```python
from build123d import *

# Parameters (mm, degrees)
F0_W     = 76.2
F0_H     = 203.2
F1_DEPTH = 6.35
F3_D     = 6.35
F5_D     = 19.05
F7_D     = 34.925


with BuildPart() as f1:
    # F0 (on Front) → F1 (new body)
    with BuildSketch(Plane.XZ):
        with Locations((38.1, 101.6)):
            Rectangle(F0_W, F0_H)
    extrude(amount=F1_DEPTH)

    # F3 (through all)
    with Locations(Plane.XZ.offset(6.35)):
        with Locations((13.868812, 74.729279), (61.493812, 74.729279), (61.493812, 27.104279), (13.868812, 27.104279)):
            Hole(F3_D / 2)

    # F5 (through all)
    with Locations(Plane.XZ.offset(6.35)):
        with Locations((38.1, 173.591416)):
            Hole(F5_D / 2)

    # F7 (through all)
    with Locations(Plane.XZ.offset(6.35)):
        with Locations((37.681312, 50.916779)):
            Hole(F7_D / 2)


solid = f1.part
```
Could you check a few things on this model? Use its own coordinates, in mm. Coordinates: 2 decimals unless noted, no trailing zeros. Write each loop counter-clockwise with the first axis right and the second up, starting at its lowest first coordinate (ties: lowest second). Pieces come first, ordered by that corner, then holes. Notation, with made-up numbers: (4.5, 69) -> (28.5, 69) arc R17 ccw to (28.5, 86) -> close; hole circle Ø6 at (-24.75, -20.75). An arc over 180 degrees is marked (long way). One line per question, with ' | ' between items. Start each with the question number.
1. Thinking about a two-plate mould opening in X: for faces 1 (the face through (0, -3, 100)), 2 (the face through (76.2, -3, 100)), 3 (the face through (51.54, -3.13, 40.29)), which applies, pulls with the +X half, pulls with the -X half, needs draft (parallel to the pull), parting line crosses it, or undercut?
2. Please list where these lines run through material, in increasing order: line 1 along Z through (x, y) = (37.5, -5.75); line 2 along Z through (x, y) = (13, -5); line 3 along X through (y, z) = (-5, 25).
3. If we section it at C-C (x = 38.1): Please give me the cut outline in (y, z), and give its area (3 significant figures).
4. If we section it at B-B (y = -5.25): Count the separate pieces of the cut face and the enclosed holes in it, and give its area (3 significant figures).
5. Will this pin go through, and if not, where does the flat tip stop? P1, Ø5, axis at x = 13.87, z = 74.73, coming from the +Y side.
6. If we section it at A-A (x = 15): Please give me the cut outline in (y, z), and give its area (3 significant figures).
Return value:
1) face 1: pulls with the -X half | face 2: pulls with the +X half | face 3: undercut
2) line 1: z = 0 to 33.46, 68.38 to 164.09, 183.1 to 203.2 | line 2: z = 0 to 24.05, 30.16 to 71.68, 77.78 to 203.2 | line 3: x = 0 to 11.49, 16.25 to 59.12, 63.87 to 76.2
3) outline: (-6.35, 0) -> (0, 0) -> (0, 33.46) -> (-6.35, 33.46) -> close; (-6.35, 68.37) -> (0, 68.37) -> (0, 164.07) -> (-6.35, 164.07) -> close; (-6.35, 183.12) -> (0, 183.12) -> (0, 203.2) -> (-6.35, 203.2) -> close | area: 948 mm²
4) separate pieces: 1 | enclosed holes: 6 | area: 14,100 mm²
5) P1: passes through
6) outline: (-6.35, 0) -> (0, 0) -> (0, 24.14) -> (-6.35, 24.14) -> close; (-6.35, 30.07) -> (0, 30.07) -> (0, 71.76) -> (-6.35, 71.76) -> close; (-6.35, 77.7) -> (0, 77.7) -> (0, 203.2) -> (-6.35, 203.2) -> close | area: 1,210 mm²
